Part print with two shaded views. Sizes in mm from the minimum x, y, z corner. Round coordinates to 2 decimals unless told otherwise and drop trailing zeros. Loops run counter-clockwise (first coordinate to the right, second up) from the corner with the lowest first, then second, coordinate; pieces in that order, holes last. Notation, with made-up numbers: M 30.5,-28 L 48.5,-28 A18 ccw 48.5,6 Z; hole C 65.5,6 d4. An arc over 180 degrees is marked long. Answer as CSV lines item,"result". Start each with the question number.
Item 1: Band-saw the part on C-C (z = 15). Give the cut face in (x, y), and give its area (3 significant figures).
Item 2: Wall check: line 1 (X direction, y = 1.75, z = 56); line 2 (Z direction, x = 194, y = 2.2); line 3 (Z direction, x = 115, y = 1.25). Give the ranges that are in metal, low to high.
Item 3: Band-saw the part on B-B (x = 221). Give the cut face in (y, z).
Item 4: Band-saw the part on A-A (y = 2.15). Count the separate pieces of the cut face and the enclosed holes in it, and give its area (3 significant figures).
Item 5: Drop flat-ended pins along their axis: pin 1 Ø1.8 at (x, z) = (135, 220) entering from -Y; pin 2 Ø1.5 at (y, z) = (2.5, 40.5) entering from +X; pin 3 Ø2.5 at (x, y) = (9, 2.5) entering from -Z. Give the stop position or say it passes through.
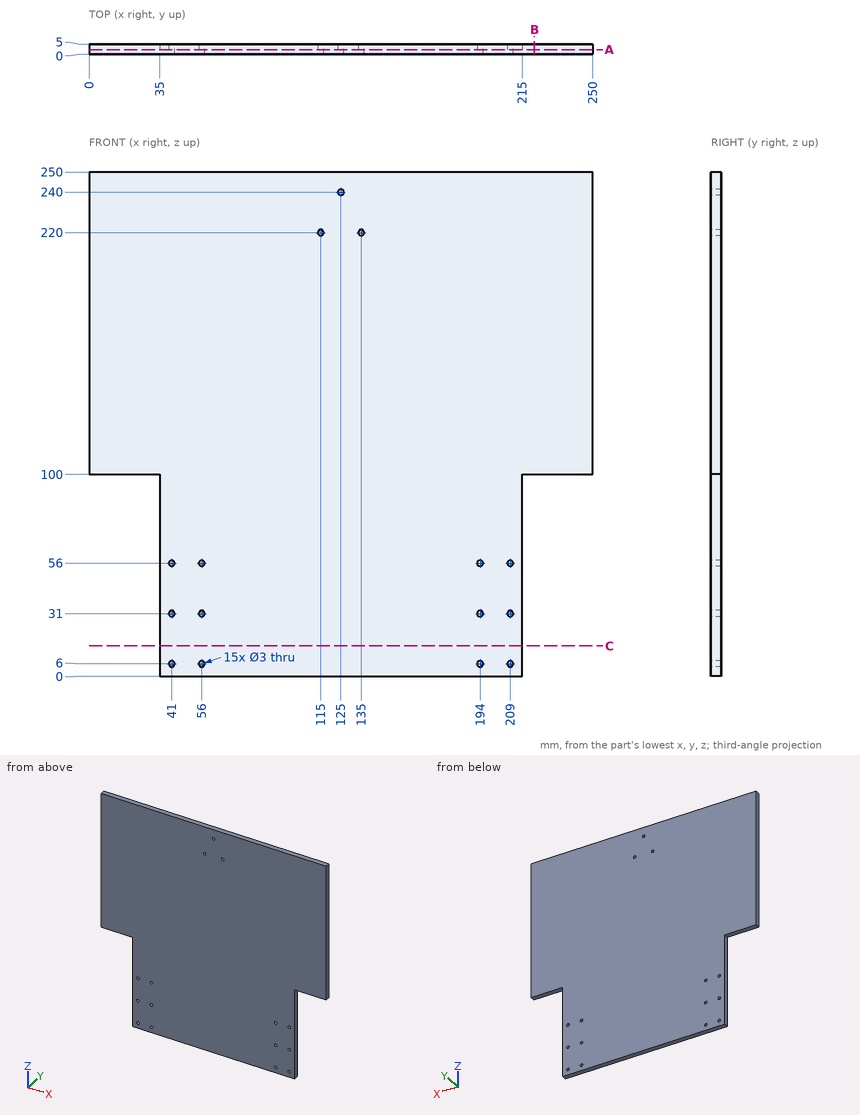
Answer block:
1,outline,"M 35,0 L 215,0 L 215,5 L 35,5 Z"
1,area,"900 mm^2"
2,line 1,"x = 35 to 39.5, 42.5 to 54.5, 57.5 to 192.5, 195.5 to 207.5, 210.5 to 215"
2,line 2,"z = 0 to 4.5, 7.5 to 29.5, 32.5 to 54.5, 57.5 to 250"
2,line 3,"z = 0 to 218.5, 221.5 to 250"
3,outline,"M 0,100 L 5,100 L 5,250 L 0,250 Z"
4,separate pieces,"1"
4,enclosed holes,"15"
4,area,"55,400 mm^2"
5,pin 1,"passes through"
5,pin 2,"stops at x = 215"
5,pin 3,"stops at z = 100"
